Design review of the part shown in the three views and the two pictorial views. Dimensions are in mm from the part's minimum x, y and z. Give positions to 0.01 mm unless a question says otherwise; leave off trailing zeros. Loops run counter-clockwise (first coordinate to the right, second up) from the corner with the lowest first, then second, coordinate; pieces in that order, holes last. Notation, with made-up numbers: (74.25, 17) - (93.25, 17) arc R32 ccw to (93.25, 44) - close; hole circle Ø5 at (86.5, 81.5). An arc over 180 degrees is marked (long way). Answer in a Markdown table with one row per item.
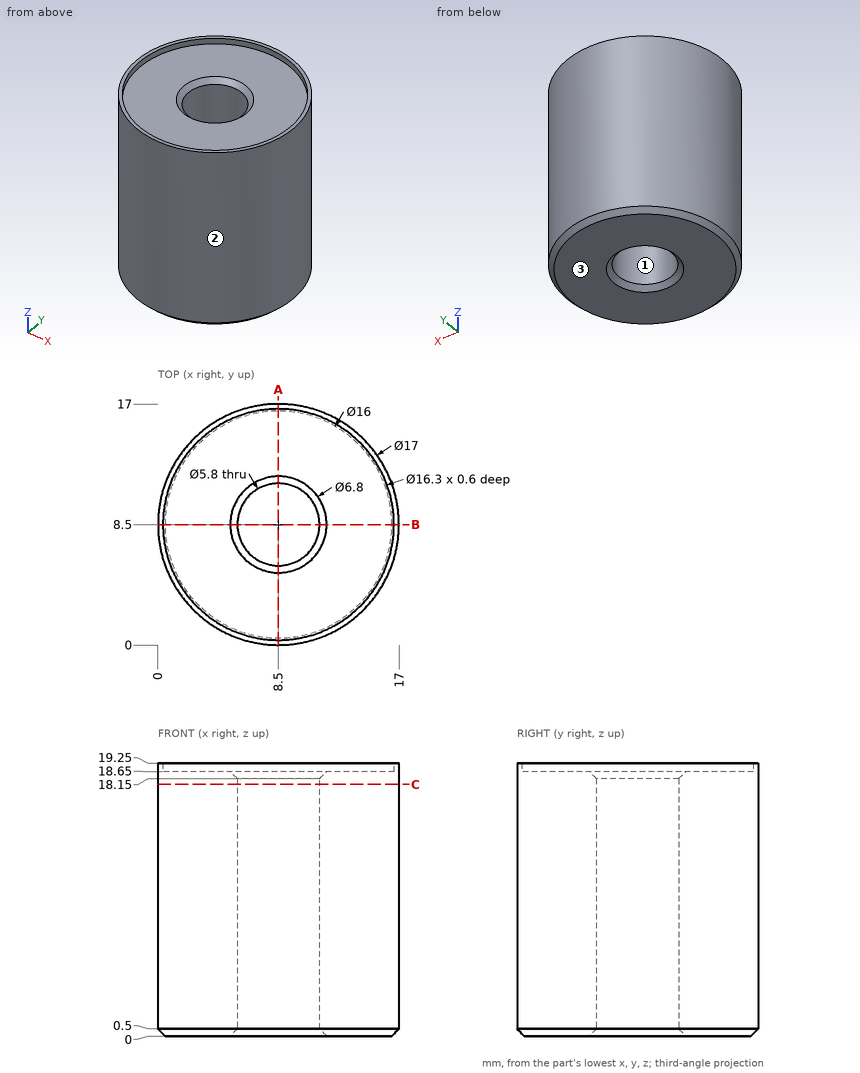
1. Mouldability with a two-part tool opening along Y and no side actions: class the marked faces 1, 2 and 3 as released by +Y, released by -Y, zero draft, split by the parting line, or undercut.
Values:
| item | result |
|---|---|
| face 1 | undercut |
| face 2 | split by the parting line |
| face 3 | zero draft |
2. Wall thickness on line 1 (Y direction, x = 8.5, z = 19.15); line 2 (Y direction, x = 8.5, z = 14.75); line 3 (Z direction, x = 4.75, y = 2.5): over which ranges is each line inside the solid? List them lowest first. Write a range as [from, to].
Values:
| item | result |
|---|---|
| line 1 | y = [0, 0.35], [16.65, 17] |
| line 2 | y = [0, 5.6], [11.4, 17] |
| line 3 | z = [0, 18.65] |
3. We need section A-A, the plane x = 8.5. Give the boundary of the cut face in (y, z), and give its area (3 significant figures).
Values:
| item | result |
|---|---|
| outline | (0, 0.5) - (0.5, 0) - (5.1, 0) - (5.6, 0.5) - (5.6, 18.15) - (5.1, 18.65) - (0.35, 18.65) - (0.35, 19.25) - (0, 19.25) - close; (11.4, 0.5) - (11.9, 0) - (16.5, 0) - (17, 0.5) - (17, 19.25) - (16.65, 19.25) - (16.65, 18.65) - (11.9, 18.65) - (11.4, 18.15) - close |
| area | 209 mm^2 |
4. Clearance check with flat-ended pins moving along their axes: pin 1 (1 mm diameter, centred on y = 10.5, z = 5.5, fed in from +X); pin 2 (6 mm diameter, centred on x = 2.5, z = 14, fed in from +Y); pin 3 (5 mm diameter, centred on y = 4, z = 14.5, fed in from +X). State where each tip first meets the part, or that it passes through.
Values:
| item | result |
|---|---|
| pin 1 | stops at x = 16.87 |
| pin 2 | stops at y = 16.45 |
| pin 3 | stops at x = 16.76 |
5. We need section C-C, the plane z = 17.75. Give the boundary of the cut face in (x, y).
Values:
| item | result |
|---|---|
| outline | circle Ø17 at (8.5, 8.5); hole circle Ø5.8 at (8.5, 8.5) |
